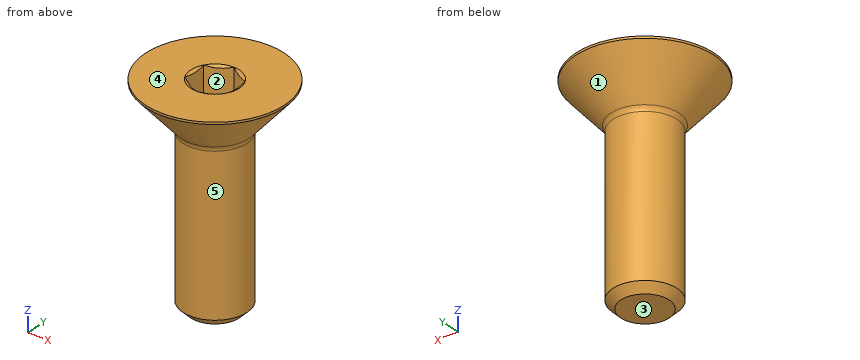
```python
from build123d import *

# Parameters (mm, degrees)
SKETCH1_W          = 15.875
SKETCH1_H          = 2.413
CHAMFER1_SIZE      = 0.5953125
CUT_EXTRUDE2_DEPTH = 2.25806


with BuildPart() as part:
    # Sketch1 → Revolve1 (revolve)
    with BuildSketch(Plane(origin=(0, 0, 0), x_dir=(0, 0, -1), z_dir=(1, 0, 0))):
        with Locations((7.9375, 1.2065)):
            Rectangle(SKETCH1_W, SKETCH1_H)
    revolve(axis=Axis((0, 0, -15.875), (0, 0, 1)))

    # Chamfer1
    chamfer1_edges = [part.edges().sort_by_distance(p)[0] for p in [
        (0, -2.413, -15.875),
    ]]
    chamfer(chamfer1_edges, length=CHAMFER1_SIZE)

    # Sketch7 → Revolve2 (revolve)
    with BuildSketch(Plane(origin=(0, 0, 0), x_dir=(0, 0, -1), z_dir=(1, 0, 0)), mode=Mode.PRIVATE) as revolve2_sk:
        with BuildLine():
            Line((0, 5.2197), (0.16129, 5.2197))
            Line((0.16129, 5.2197), (3.2258, 2.555762099))
            ThreePointArc((3.2258, 2.555762099), (3.403809493, 2.44985758), (3.607634579, 2.413))
            Line((3.607634579, 2.413), (3.607634579, 0))
            Line((3.607634579, 0), (0, 0))
            Line((0, 0), (0, 5.2197))
        make_face()
    revolve(revolve2_sk.sketch.rotate(Axis((0, 0, 0), (0, 0, -1)), 180), axis=Axis((0, 0, 0), (0, 0, -1)))

    # Sketch5 → Cut-Extrude2 (cut)
    with BuildSketch(Plane.XY):
        Polygon((0, 1.833087105), (-1.5875, 0.916543552), (-1.5875, -0.916543552), (0, -1.833087105), (1.5875, -0.916543552), (1.5875, 0.916543552), align=None)
    extrude(amount=-CUT_EXTRUDE2_DEPTH, mode=Mode.SUBTRACT)

    # Cut-Extrude3 cone 1 section (through the dimple's axis) → Cut-Extrude3 (revolve, cut)
    with BuildSketch(Plane(origin=(0, 0, 0), x_dir=(0, -1, 0), z_dir=(1, 0, 0))):
        Polygon((0, 0), (1.833087105, 0), (0, 1.058333333), align=None)
    revolve(axis=Axis((0, 0, 0), (0, 0, -1)), mode=Mode.SUBTRACT)


solid = part.part
```
Work out the finished part from the listing and answer in its coordinate system (mm). Face numbers are marked on the shaded views. A direction names the side the tool comes from. Give positions to 0.01 mm unless a question says otherwise; leave off trailing zeros. Loops run counter-clockwise (first coordinate to the right, second up) from the corner with the lowest first, then second, coordinate; pieces in that order, holes last. Notation, with made-up numbers: (20.5, -34.5) - (77.5, -34.5) arc R27 cw to (77.5, -11.5) - close; hole circle Ø11 at (45.25, -9.5). An arc over 180 degrees is marked (long way). Use CSV: the item, a comma, the result in double quotes. Start each with the question number.
(1) Find section B-B, the plane z = -10.75. Determine the outline of the cut face in (x, y), plus the area to 3 significant figures.
(2) Find the intervals of material crossed by L1, parallel to Z at x = 1.25, y = 0.25 (3 decimals); L2, parallel to Y at x = -0.5, z = -1.75; L3, parallel to X at y = 0, z = -10.75, in increasing order.
(3) A tool of negligible diameter and unlimited length cuts with its end or side. For the marked faces 4 and 5, from which of +Z, -Z, +X, -X, +Y, -Y can it reach the whole face along a straight path? Write none if from no direction.
(4) Each of these flat-tipped pins is pushed along its axis until it touches: pin 1 (6 mm diameter, centred on y = 0, z = -8.5, fed in from -X); pin 2 (2 mm diameter, centred on x = 3.5, z = -13.5, fed in from -Y); pin 3 (4 mm diameter, centred on x = -3.5, z = -12.5, fed in from -Y); pin 4 (0.9 mm diameter, centred on y = 0.5, z = -1, fed in from +X). Where does it stop, or does it pass through?
(5) Determine the mould class of the marked faces 1, 2 and 3 for opening direction Y: released by +Y, released by -Y, zero draft, split by the parting line, or undercut.
Results found:
1,outline,"circle Ø4.83 at (0, 0)"
1,area,"18.3 mm^2"
2,L1,"-15.875 to -2.258"
2,L2,"-3.81 to -1.54, 1.54 to 3.81"
2,L3,"-2.41 to 2.41"
3,face 4,"+Z, +X, -X, +Y, -Y"
3,face 5,"-Z"
4,pin 1,"x = -2.41"
4,pin 2,"through"
4,pin 3,"y = -1.89"
4,pin 4,"x = 4.86"
5,face 1,"split by the parting line"
5,face 2,"undercut"
5,face 3,"zero draft"
